```python
from build123d import *

# Parameters (mm, degrees)
SKETCH1_W           = 46
SKETCH1_H           = 46
BOSS_EXTRUDE1_DEPTH = 80
CUT_EXTRUDE1_DEPTH  = 20
SKETCH3_R           = 5
CUT_EXTRUDE2_DEPTH  = 21
SKETCH4_R           = 5
CUT_EXTRUDE3_DEPTH  = 21
SKETCH5_R           = 2.75
CUT_EXTRUDE4_DEPTH  = 47
SKETCH6_R           = 2.75
CUT_EXTRUDE5_DEPTH  = 47
FILLET1_R           = 5
SKETCH9_R           = 2.75
CUT_EXTRUDE8_DEPTH  = 81
SKETCH10_R          = 2.75
CUT_EXTRUDE9_DEPTH  = 61
SKETCH11_R          = 5
CUT_EXTRUDE10_DEPTH = 55


with BuildPart() as part:
    # Sketch1 → Boss-Extrude1 (new body)
    with BuildSketch(Plane(origin=(0, 0, 0), x_dir=(1, 0, 0), z_dir=(0, 1, 0))):
        with Locations((23, 23)):
            Rectangle(SKETCH1_W, SKETCH1_H)
    extrude(amount=BOSS_EXTRUDE1_DEPTH)

    # Sketch2 → Cut-Extrude1 (cut)
    with BuildSketch(Plane(origin=(0, 80, 0), x_dir=(1, 0, 0), z_dir=(0, 1, 0))):
        Polygon((0, 46), (20, 46), (20, 20), (46, 20), (46, 0), (20, 0), (0, 0), align=None)
    extrude(amount=-CUT_EXTRUDE1_DEPTH, mode=Mode.SUBTRACT)

    # Sketch3 → Cut-Extrude2 (cut)
    with BuildSketch(Plane(origin=(46, 0, 0), x_dir=(0, 0, -1), z_dir=(1, 0, 0))):
        with Locations((33, 70)):
            Circle(SKETCH3_R)
    extrude(amount=-CUT_EXTRUDE2_DEPTH, mode=Mode.SUBTRACT)

    # Sketch4 → Cut-Extrude3 (cut)
    with BuildSketch(Plane(origin=(0, 0, -46), x_dir=(-1, 0, 0), z_dir=(0, 0, -1))):
        with Locations((-33, 70)):
            Circle(SKETCH4_R)
    extrude(amount=-CUT_EXTRUDE3_DEPTH, mode=Mode.SUBTRACT)

    # Sketch5 → Cut-Extrude4 (cut, through all)
    with BuildSketch(Plane(origin=(0, 0, -46), x_dir=(-1, 0, 0), z_dir=(0, 0, -1))):
        with Locations((-33, 70)):
            Circle(SKETCH5_R)
    extrude(amount=-CUT_EXTRUDE4_DEPTH, mode=Mode.SUBTRACT)

    # Sketch6 → Cut-Extrude5 (cut, through all)
    with BuildSketch(Plane(origin=(46, 0, 0), x_dir=(0, 0, -1), z_dir=(1, 0, 0))):
        with Locations((33, 70)):
            Circle(SKETCH6_R)
    extrude(amount=-CUT_EXTRUDE5_DEPTH, mode=Mode.SUBTRACT)

    # Fillet1
    fillet1_edges = [part.edges().sort_by_distance(p)[0] for p in [
        (0, 30, -46),
        (46, 30, 0),
        (0, 30, 0),
        (46, 40, -46),
    ]]
    fillet(fillet1_edges, radius=FILLET1_R)

    # Sketch9 → Cut-Extrude8 (cut, through all)
    with BuildSketch(Plane.XZ):
        with Locations((10, -33)):
            Circle(SKETCH9_R)
    extrude(amount=-CUT_EXTRUDE8_DEPTH, mode=Mode.SUBTRACT)

    # Sketch10 → Cut-Extrude9 (cut, through all)
    with BuildSketch(Plane(origin=(0, 60, 0), x_dir=(1, 0, 0), z_dir=(0, 1, 0))):
        with Locations((33, 10)):
            Circle(SKETCH10_R)
    extrude(amount=-CUT_EXTRUDE9_DEPTH, mode=Mode.SUBTRACT)

    # Sketch11 → Cut-Extrude10 (cut)
    with BuildSketch(Plane.XZ):
        with Locations((33, -10)):
            Circle(SKETCH11_R)
        with Locations((10, -33)):
            Circle(SKETCH11_R)
    extrude(amount=-CUT_EXTRUDE10_DEPTH, mode=Mode.SUBTRACT)


solid = part.part
```
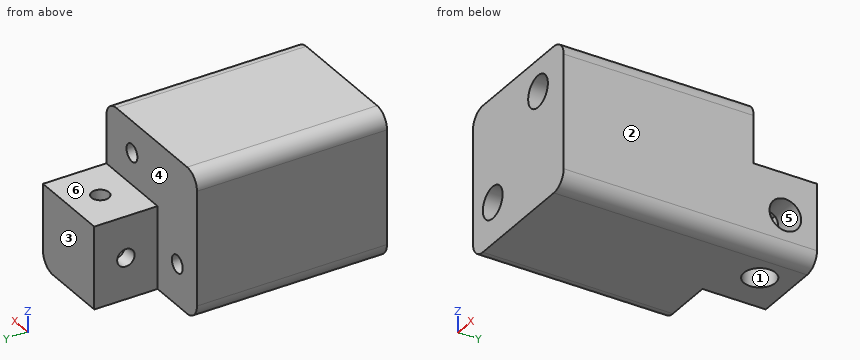
Read the model definition and answer for the solid it produces. Units are mm, in the model's axes. Face numbers are marked on the shaded views. A direction names the side the tool comes from. Coordinates: 2 decimals unless noted, no trailing zeros. Loops run counter-clockwise (first coordinate to the right, second up) from the corner with the lowest first, then second, coordinate; pieces in that order, holes last.
(1) The mould has two halves that part along Y. Classify the marked faces 1, 2 and 3: released by +Y, released by -Y, zero draft, split by the parting line, or undercut.
Solution:
face 1: undercut
face 2: zero draft
face 3: released by +Y
(2) Consider line 1 along Y through (x, z) = (33, -28.5); line 2 along Y through (x, z) = (21, -33); line 3 along Z through (x, y) = (10, 57). Determine where each line is inside the solid, lowest interval first.
Solution:
line 1: y = 0 to 65, 75 to 80
line 2: y = 0 to 67.25, 72.75 to 80
line 3: z = -46 to -35.75, -30.25 to 0
(3) The part is cut by section C-C (z = -40). Determine the outline of the cut face in (x, y).
Solution:
outline: (0, 0) - (46, 0) - (46, 80) - (20, 80) - (20, 60) - (0, 60) - close; hole circle Ø10 at (33, 70)
(4) A tool of negligible diameter and unlimited length cuts with its end or side. For the marked faces 4, 5 and 6, from which of +Z, -Z, +X, -X, +Y, -Y can it reach the whole face along a straight path? Write none if from no direction.
Solution:
face 4: +Z, -X, +Y
face 5: +X
face 6: +Z, +X, -X, +Y
(5) Flat-ended cylindrical pins translate along their axes: pin 1 Ø7 at (x, y) = (33, 70) entering from +Z; pin 2 Ø6 at (y, z) = (67.5, -30.5) entering from -X; pin 3 Ø9 at (x, y) = (33, 70) entering from -Z; pin 4 Ø3 at (x, z) = (6.5, -36) entering from -Y. Find the tip coordinate at first contact, or state that the pin passes through.
Solution:
pin 1: stops at z = -20
pin 2: stops at x = 20
pin 3: stops at z = -25
pin 4: stops at y = 0
(6) The part is cut by section D-D (x = 40). Determine the outline of the cut face in (y, z), and give its area (3 significant figures).
Solution:
outline: (0, -46) - (80, -46) - (80, -20) - (60, -20) - (60, 0) - (0, 0) - close; hole circle Ø10 at (70, -33)
area: 3,200 mm2
(7) The part is cut by section A-A (x = 10). Determine the outline of the cut face in (y, z), and give its area (3 significant figures).
Solution:
outline: (0, -46) - (60, -46) - (60, -35.75) - (55, -35.75) - (55, -38) - (0, -38) - close; (0, -28) - (55, -28) - (55, -30.25) - (60, -30.25) - (60, 0) - (0, 0) - close
area: 2,180 mm2
(8) The part is cut by section B-B (y = 70). Determine the outline of the cut face in (x, z), and give its area (3 significant figures).
Solution:
outline: (20, -46) - (28, -46) - (28, -38) - (25, -38) - (25, -35.75) - (20, -35.75) - close; (20, -30.25) - (25, -30.25) - (25, -28) - (28, -28) - (28, -25) - (30.25, -25) - (30.25, -20) - (20, -20) - close; (35.75, -25) - (38, -25) - (38, -28) - (46, -28) - (46, -20) - (35.75, -20) - close; (38, -46) - (41, -46) arc R5 ccw to (46, -41) - (46, -38) - (38, -38) - close
area: 296 mm2
